Geometry: final body of the model. Coordinates: model frame, mm. Face numbers are marked on the shaded views. Coordinates: 2 decimals unless noted, no trailing zeros. Order: outer loops, then holes, each group sorted by start corner. A loop starts at its lowest first (then second) coordinate and runs counter-clockwise, first axis right, second up. Notation, with made-up numbers: M -24.5,78.25 L 21.5,78.25 A36 cw 21.5,113.25 Z; hole C -17.75,38 d7. An arc over 180 degrees is marked long. Write item = value, one per line. Start each with the question number.
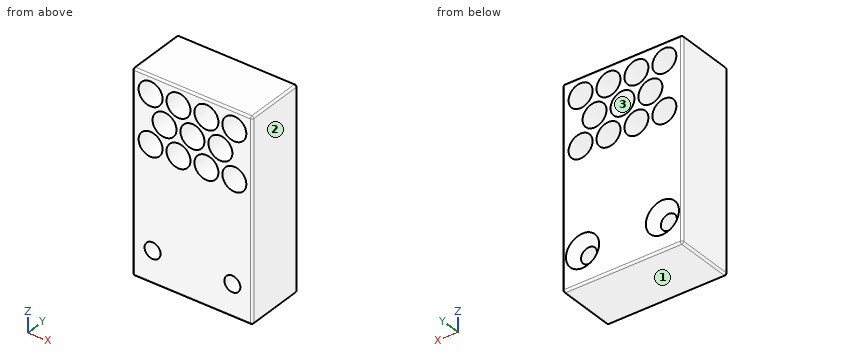
Autodesk Inventor part; units mm, degrees
ref_plane "YZ Plane" through (0, 0, 0) normal (1, 0, 0) x (0, 1, 0)
ref_plane "XZ Plane" through (0, 0, 0) normal (0, 1, 0) x (-1, 0, 0)
ref_plane "XY Plane" through (0, 0, 0) normal (0, 0, 1) x (1, 0, 0)
sketch "Skizze1" plane through (0, 0, 0) normal (0, 1, 0) x (-1, 0, 0)
  line L0 (-24.6188, -3.2813) -> (5.3812, -3.2813)
  line L1 (5.3812, -3.2813) -> (5.3812, 46.7188)
  line L2 (5.3812, 46.7188) -> (-24.6188, 46.7188)
  line L3 (-24.6188, 46.7188) -> (-24.6188, -3.2813)
  line L4 (-24.6188, -3.2813) -> (5.3812, 46.7188) construction
  line L5 (5.3812, -3.2813) -> (-24.6188, 46.7188) construction
  point P0 (0, 0)
  point P1 (-9.6188, 21.7188)
  dimension "d5" = 50
  dimension "d7" = 30
extrude "Extrusion1" add sketch "Skizze1" along normal blind 15
fillet "Rundung1" radius 0.5 12 edges at (24.6188, 7.5, 46.7188) (24.6188, 7.5, -3.2813) (24.6188, 0, 21.7188) (24.6188, 15, 21.7188) (-5.3812, 7.5, 46.7188) (9.6188, 0, 46.7188) (9.6188, 15, 46.7188) (-5.3812, 7.5, -3.2813) (-5.3812, 0, 21.7187) (-5.3812, 15, 21.7187) (9.6188, 0, -3.2813) (9.6188, 15, -3.2813)
sketch "Skizze2" plane through (-4.8812, 15, -2.7813) normal (0, 1, 0) x (1, 0, 0)
  line L0 (29, -49) -> (0, -49)
  circle A0 centre (25, -45) radius 3
  circle A1 centre (21.5, -38.9378) radius 3
  line L1 (29.5, -49) -> (29.5, 0) construction
  line L2 (0, -49.5) -> (29, -49.5) construction
  circle A2 centre (18, -45) radius 3
  circle A3 centre (11, -45) radius 3
  circle A4 centre (4, -45) radius 3
  circle A5 centre (25, -32.8756) radius 3
  circle A6 centre (14.5, -38.9378) radius 3
  circle A7 centre (7.5, -38.9378) radius 3
  circle A8 centre (18, -32.8756) radius 3
  circle A9 centre (11, -32.8756) radius 3
  circle A10 centre (4, -32.8756) radius 3
  point P0 (4.8812, -2.7813)
  dimension "d9" = 6
  dimension "d66" = 7
  dimension "d81" = 4.5
  dimension "d82" = 4.5
  dimension "d86" = 7
  dimension "d93" = 7
  dimension "d112" = 0
  dimension "d113" = 1
  dimension "d115" = 1
  dimension "d116" = 1
  dimension "d117" = 6.0622
extrude "Extrusion2" cut sketch "Skizze2" against normal through all
sketch "Skizze3" plane through (0, 15, 0) normal (0, 1, 0) x (1, 0, 0)
  circle A0 centre (-0.3812, -4.7187) radius 2
  circle A1 centre (19.6188, -4.7187) radius 2
  line L0 (24.1188, 3.2813) -> (-4.8812, 3.2813)
  line L1 (24.6188, -46.2187) -> (24.6188, 2.7813)
  line L2 (-5.3812, 2.7813) -> (-5.3812, -46.2188)
  point P0 (0, 0)
  dimension "d40" = 4
  dimension "d43" = 4
  dimension "d105" = 8
  dimension "d106" = 8
  dimension "d107" = 5
  dimension "d108" = 5
  dimension "d118" = 20
hole "Bohrung1" at (-0.3812, 15, 4.7187) at (19.6188, 15, 4.7187) direction (0, -1, 0) diameter 4 end through all countersink diameter 8.3 countersink angle 90
properties part number "Schlauchhalter"
Item 1: Material intervals for probe 1 along X at (y, z) = (5, 31); probe 2 along X at (y, z) = (0.75, 5.5); probe 3 along X at (y, z) = (3.5, 6), sorted ascending. Write a range as [from, to].
Item 2: Section query B-B on z = 29. Output: boundary loops of the cut face in (x, y), and give its area (3 significant figures).
Item 3: Section query A-A on z = 35. Output: boundary loops of the cut face in (x, y), and give its area (3 significant figures).
Item 4: Section query C-C on y = 2.25. Give the number of separate pieces and of enclosed holes in the cut face, and give its area (3 significant figures).
Item 5: First-contact query: pin 1 (3.5 mm diameter, centred on x = -0.88, z = 42.22, fed in from -Y). Flat tip, straight axial feed; report the tip coordinate or a pass-through.
Item 6: Draft query along X for the marked faces 1, 2 and 3. Return one class per face: pulls with the +X half, pulls with the -X half, needs draft (parallel to the pull), parting line crosses it, or undercut.
Ans:
q1.probe_1 = [-5.38, -3.74], [1.98, 3.26], [8.98, 10.26], [15.98, 17.26], [22.98, 24.62]
q1.probe_2 = [-5.38, -2.22], [1.46, 17.78], [21.46, 24.62]
q1.probe_3 = [-5.38, -1.92], [1.15, 18.08], [21.15, 24.62]
q2.outline = M -5.38,0.5 A0.5 ccw -4.88,0 L -3.67,0 L -3.67,15 L -4.88,15 A0.5 ccw -5.38,14.5 Z; M 1.91,0 L 3.33,0 L 3.33,15 L 1.91,15 Z; M 8.91,0 L 10.33,0 L 10.33,15 L 8.91,15 Z; M 15.91,0 L 17.33,0 L 17.33,15 L 15.91,15 Z; M 22.91,0 L 24.12,0 A0.5 ccw 24.62,0.5 L 24.62,14.5 A0.5 ccw 24.12,15 L 22.91,15 Z
q2.area = 115 mm^2
q3.outline = M -5.38,0.5 A0.5 ccw -4.88,0 L -0.15,0 L -0.15,15 L -4.88,15 A0.5 ccw -5.38,14.5 Z; M 5.39,0 L 6.85,0 L 6.85,15 L 5.39,15 Z; M 12.39,0 L 13.85,0 L 13.85,15 L 12.39,15 Z; M 19.39,0 L 24.12,0 A0.5 ccw 24.62,0.5 L 24.62,14.5 A0.5 ccw 24.12,15 L 19.39,15 Z
q3.area = 201 mm^2
q4.separate_pieces = 1
q4.enclosed_holes = 13
q4.area = 1,160 mm^2
q5.pin_1 = through
q6.face_1 = needs draft
q6.face_2 = pulls with the +X half
q6.face_3 = undercut
